Geometry: final body of the model. Coordinates: model frame, mm. A direction names the side the tool comes from. Give positions to 0.01 mm unless a question says otherwise; leave off trailing zeros. Loops run counter-clockwise (first coordinate to the right, second up) from the corner with the lowest first, then second, coordinate; pieces in that order, holes last.
1. Section A-A, the plane z = -8.5. State how many separate pieces and enclosed holes the cut face has, then the cut area to 3 significant figures.
2. Access query for faces 1 (the face through (-5650, 1537.97, -6)), 2 (the face through (-5363, 1518, -3.175)), 3 (the face through (-5278, 1384.3, -6)), 4 (the face through (-5374, 1550.67, -6)), 5 (the face through (-5099, 1537.97, -6)). Directions: +Z, -Z, +X, -X, +Y, -Y. A direction counts if a zero-diameter tool reaches every point of the face in a straight line with its end or side. Return the directions, or none.
3. Section B-B, the plane y = 1481. Output: boundary loops of the cut face in (x, z) (1 decimal), then the cut area to 3 significant figures.
4. Draft query along X for faces 6 (the face through (-5740.4, 1457, -6)), 7 (the face through (-5381, 1532, -12.7)), 8 (the face through (-5475, 1384.3, -6)). Return one class per face: +X half, -X half, draft (parallel to the pull), parting line (faces both ways), or undercut.
5. Material intervals for line 1 along X through (y, z) = (1409.7, -10) (1 decimal); line 2 along X through (y, z) = (1444, -4.75) (1 decimal); line 3 along X through (y, z) = (1476.5, -3), sorted ascending.
6. First-contact query: P1, Ø2, axis at x = -5362.5, z = -8.5, coming from the -Y side; P2, Ø4, axis at y = 1548.5, z = -9.5, coming from the +X side; P3, Ø6.5, axis at x = -5199.5, z = -9, coming from the -Y side (3 decimals). Flat tips, straight axial feed; report the tip coordinate or a pass-through.
7. Section D-D, the plane x = -5485.5. Output: boundary loops of the cut face in (y, z) (3 decimals).
from build123d import *

# Parameters (mm, degrees)
EXTRUDE1_DEPTH     = 12.7
SKETCH6_R          = 3.302
CUT_EXTRUDE4_DEPTH = 12.7
CUT_EXTRUDE1_DEPTH = 3.175
SKETCH4_R          = 1.5875
CUT_EXTRUDE2_DEPTH = 12.7
SKETCH5_W          = 363.5375
SKETCH5_H          = 6.35
CUT_EXTRUDE3_DEPTH = 6.35
SKETCH7_W          = 101.6
SKETCH7_H          = 5.08
EXTRUDE2_DEPTH     = 12.7
SKETCH8_R          = 3.175
CUT_EXTRUDE5_DEPTH = 12.7


with BuildPart() as part:
    # Sketch2 → Extrude1 (new body)
    with BuildSketch(Plane.XY):
        with BuildLine():
            Line((-5740.4, 1537.97), (-5740.4, 1384.3))
            Line((-5740.4, 1384.3), (-5584.03125, 1384.3))
            Line((-5584.03125, 1384.3), (-5584.03125, 1392.2375))
            ThreePointArc((-5584.03125, 1392.2375), (-5581.706410076, 1397.850160076), (-5576.09375, 1400.175))
            Line((-5576.09375, 1400.175), (-5506.24375, 1400.175))
            ThreePointArc((-5506.24375, 1400.175), (-5500.631089924, 1397.850160076), (-5498.30625, 1392.2375))
            Line((-5498.30625, 1392.2375), (-5498.30625, 1384.3))
            Line((-5498.30625, 1384.3), (-5451.475, 1384.3))
            Line((-5451.475, 1384.3), (-5451.475, 1512.8875))
            ThreePointArc((-5451.475, 1512.8875), (-5450.54506403, 1515.13256403), (-5448.3, 1516.0625))
            Line((-5448.3, 1516.0625), (-5303.8375, 1516.0625))
            ThreePointArc((-5303.8375, 1516.0625), (-5301.59243597, 1515.13256403), (-5300.6625, 1512.8875))
            Line((-5300.6625, 1512.8875), (-5300.6625, 1384.3))
            Line((-5300.6625, 1384.3), (-5253.83125, 1384.3))
            Line((-5253.83125, 1384.3), (-5253.83125, 1392.2375))
            ThreePointArc((-5253.83125, 1392.2375), (-5251.506410076, 1397.850160076), (-5245.89375, 1400.175))
            Line((-5245.89375, 1400.175), (-5176.04375, 1400.175))
            ThreePointArc((-5176.04375, 1400.175), (-5170.431089924, 1397.850160076), (-5168.10625, 1392.2375))
            Line((-5168.10625, 1392.2375), (-5168.10625, 1384.3))
            Line((-5168.10625, 1384.3), (-5011.7375, 1384.3))
            Line((-5011.7375, 1384.3), (-5011.7375, 1537.97))
            Line((-5011.7375, 1537.97), (-5194.3, 1537.97))
            Line((-5194.3, 1537.97), (-5194.3, 1550.67))
            Line((-5194.3, 1550.67), (-5557.8375, 1550.67))
            Line((-5557.8375, 1550.67), (-5557.8375, 1537.97))
            Line((-5557.8375, 1537.97), (-5740.4, 1537.97))
        make_face()
    extrude(amount=-EXTRUDE1_DEPTH)

    # Sketch6 → Cut-Extrude4 (cut)
    with BuildSketch(Plane.XY):
        with Locations((-5560.08256403, 1540.21506403)):
            Circle(SKETCH6_R)
        with Locations((-5192.05493597, 1540.21506403)):
            Circle(SKETCH6_R)
    extrude(amount=-CUT_EXTRUDE4_DEPTH, mode=Mode.SUBTRACT)

    # Sketch3 → Cut-Extrude1 (cut)
    with BuildSketch(Plane.XY):
        with BuildLine():
            Line((-5297.4875, 1377.95), (-5454.65, 1377.95))
            ThreePointArc((-5454.65, 1377.95), (-5459.140128061, 1379.809871939), (-5461, 1384.3))
            Line((-5461, 1384.3), (-5461, 1516.0625))
            ThreePointArc((-5461, 1516.0625), (-5458.210192091, 1522.797692091), (-5451.475, 1525.5875))
            Line((-5451.475, 1525.5875), (-5300.6625, 1525.5875))
            ThreePointArc((-5300.6625, 1525.5875), (-5293.927307909, 1522.797692091), (-5291.1375, 1516.0625))
            Line((-5291.1375, 1516.0625), (-5291.1375, 1384.3))
            ThreePointArc((-5291.1375, 1384.3), (-5292.997371939, 1379.809871939), (-5297.4875, 1377.95))
        make_face()
    extrude(amount=-CUT_EXTRUDE1_DEPTH, mode=Mode.SUBTRACT)

    # Sketch4 → Cut-Extrude2 (cut)
    with BuildSketch(Plane.XY):
        with Locations((-5734.05, 1511.3)):
            Circle(SKETCH4_R)
        with Locations((-5734.05, 1409.7)):
            Circle(SKETCH4_R)
        with Locations((-5018.0875, 1409.7)):
            Circle(SKETCH4_R)
        with Locations((-5018.0875, 1511.3)):
            Circle(SKETCH4_R)
    extrude(amount=-CUT_EXTRUDE2_DEPTH, mode=Mode.SUBTRACT)

    # Sketch5 → Cut-Extrude3 (cut)
    with BuildSketch(Plane(origin=(0, 0, -12.7), x_dir=(-1, 0, 0), z_dir=(0, 0, -1))):
        with Locations((5376.06875, 1543.05)):
            Rectangle(SKETCH5_W, SKETCH5_H)
    extrude(amount=-CUT_EXTRUDE3_DEPTH, mode=Mode.SUBTRACT)

    # Sketch7 → Extrude2 (add)
    with BuildSketch(Plane.XY):
        with Locations((-5689.6, 1381.76)):
            Rectangle(SKETCH7_W, SKETCH7_H)
        with Locations((-5062.5375, 1381.76)):
            Rectangle(SKETCH7_W, SKETCH7_H)
    extrude(amount=-EXTRUDE2_DEPTH)

    # Sketch8 → Cut-Extrude5 (cut)
    with BuildSketch(Plane.XY):
        with Locations((-5635.625, 1384.3)):
            Circle(SKETCH8_R)
        with Locations((-5116.5125, 1384.3)):
            Circle(SKETCH8_R)
    extrude(amount=-CUT_EXTRUDE5_DEPTH, mode=Mode.SUBTRACT)


solid = part.part
Answers below:
1. separate pieces: 2
1. enclosed holes: 4
1. area: 92,700 mm2
2. face 1: +Z, -Z, -X, +Y
2. face 2: +Z, -Y
2. face 3: +Z, -Z, -Y
2. face 4: +Z, -Z, +X, -X, +Y
2. face 5: +Z, -Z, +X, +Y
3. outline: (-5740.4, -12.7) - (-5451.5, -12.7) - (-5451.5, -3.2) - (-5461, -3.2) - (-5461, 0) - (-5740.4, 0) - close; (-5300.7, -12.7) - (-5011.7, -12.7) - (-5011.7, 0) - (-5291.1, 0) - (-5291.1, -3.2) - (-5300.7, -3.2) - close
3. area: 7,280 mm2
4. face 6: -X half
4. face 7: draft
4. face 8: undercut
5. line 1: x = -5740.4 to -5735.6, -5732.5 to -5451.5, -5300.7 to -5019.7, -5016.5 to -5011.7
5. line 2: x = -5740.4 to -5451.5, -5300.7 to -5011.7
5. line 3: x = -5740.4 to -5461, -5291.14 to -5011.74
6. P1: stops at y = 1516.06
6. P2: stops at x = -5194.3
6. P3: stops at y = 1400.175
7. outline: (1384.3, -12.7) - (1539.875, -12.7) - (1539.875, -6.35) - (1546.225, -6.35) - (1546.225, -12.7) - (1550.67, -12.7) - (1550.67, 0) - (1384.3, 0) - close
